```python
from build123d import *

# Parameters (mm, degrees)
HOLE1_D           = 2.7178
HOLE1_DEPTH       = 8.636
HOLE1_CSINK_D     = 2.9972
HOLE1_CSINK_ANGLE = 60
HOLE1_TIP         = 0.816509495


with BuildPart() as part:
    # Sketch1 → RevolutionAngle1 (revolve)
    with BuildSketch(Plane.XY, mode=Mode.PRIVATE) as revolutionangle1_sk:
        with BuildLine():
            Line((0.127, 1.8161), (1.3462, 1.8161))
            Line((1.3462, 1.8161), (1.3462, 2.3749))
            Line((1.3462, 2.3749), (2.54, 2.3749))
            Line((2.54, 2.3749), (2.54, 1.8034))
            Line((2.54, 1.8034), (10.2108, 1.8034))
            Line((10.2108, 1.8034), (10.4648, 1.5494))
            Line((10.4648, 1.5494), (10.4648, 0))
            Line((10.4648, 0), (0, 0))
            Line((0, 0), (0, 1.6891))
            ThreePointArc((0, 1.6891), (0.037197439, 1.778902561), (0.127, 1.8161))
        make_face()
    revolve(revolutionangle1_sk.sketch.rotate(Axis((0, 0, 0), (1, 0, 0)), 90), axis=Axis((0, 0, 0), (1, 0, 0)))

    # Hole1
    with Locations(Plane.ZY):
        with Locations((0, 0)):
            CounterSinkHole(HOLE1_D / 2, HOLE1_CSINK_D / 2, depth=HOLE1_DEPTH, counter_sink_angle=HOLE1_CSINK_ANGLE)
            with Locations((0, 0, -(HOLE1_DEPTH + HOLE1_TIP / 2))):  # 118° drill point
                Cone(0, HOLE1_D / 2, HOLE1_TIP, mode=Mode.SUBTRACT)


solid = part.part
```
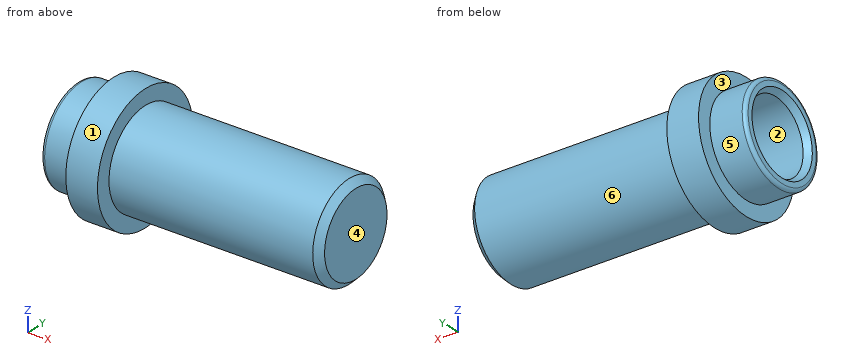
For this review, take the finished solid that the model builds, in its own axes (mm). Face numbers are marked on the shaded views. A direction names the side the tool comes from. Coordinates: 2 decimals unless noted, no trailing zeros. Loops run counter-clockwise (first coordinate to the right, second up) from the corner with the lowest first, then second, coordinate; pieces in that order, holes last.
1. Add section B-B, the plane y = 2.05. Give the boundary of the cut face in (x, z).
2. Mouldability with a two-part tool opening along Y and no side actions: class the marked faces 1, 2 and 3 as +Y half, -Y half, draft (parallel to the pull), parting line (faces both ways), or undercut.
3. For line 1 (Y direction, x = 4, z = 0); line 2 (X direction, y = -2.1, z = -0.1); line 3 (Y direction, x = 8.25, z = 0.9), list the stretches that pass through material, from the lowest coordinate up.
4. For the marked faces 4, 5 and 6, list the 3-axis set-ups (+Z, -Z, +X, -X, +Y, -Y) from which the entire face can be reached by the end or side of a thin tool; tool diameter is ignored.
5. Add section A-A, the plane x = 6.5. Give the boundary of the cut face in (y, z).
6. Insertion check: P1, Ø1.5, axis at y = 0.5, z = 0, coming from the -X side; P2, Ø1, axis at x = 2, z = -2, coming from the +Y side; P3, Ø2, axis at x = 4, z = -2, coming from the -Y side; P4, Ø2, axis at x = 2.5, y = -0.5, coming from the +Z side. Each pin has a flat end and moves straight along its axis. Give the tip position at first contact, or say it passes through.
Result:
1. outline: (1.35, -1.2) - (2.54, -1.2) - (2.54, 1.2) - (1.35, 1.2) - close
2. face 1: parting line
2. face 2: undercut
2. face 3: draft
3. line 1: y = -1.8 to -1.36, 1.36 to 1.8
3. line 2: x = 1.35 to 2.54
3. line 3: y = -1.56 to -1.02, 1.02 to 1.56
4. face 4: +Z, -Z, +X, +Y, -Y
4. face 5: -X
4. face 6: +X
5. outline: circle Ø3.61 at (0, 0); hole circle Ø2.72 at (0, 0)
6. P1: stops at x = 8.7
6. P2: stops at y = 1.84
6. P3: stops at y = -1.5
6. P4: stops at z = 2.37
